Autodesk Inventor part; units mm, degrees
ref_plane "YZ Plane" through (0, 0, 0) normal (1, 0, 0) x (0, 1, 0)
ref_plane "XZ Plane" through (0, 0, 0) normal (0, 1, 0) x (-1, 0, 0)
ref_plane "XY Plane" through (0, 0, 0) normal (0, 0, 1) x (1, 0, 0)
sketch "Boceto1" plane through (0, 0, 0) normal (0, 0, 1) x (1, 0, 0)
  line L0 (-9.55, -9.55) -> (9.55, -9.55)
  line L1 (9.55, -9.55) -> (9.55, 9.55)
  line L2 (9.55, 9.55) -> (-9.55, 9.55)
  line L3 (-9.55, 9.55) -> (-9.55, -9.55)
  line L4 (-9.55, -9.55) -> (9.55, 9.55) construction
  line L5 (9.55, -9.55) -> (-9.55, 9.55) construction
  line L6 (-8.55, 8.55) -> (8.55, 8.55)
  line L7 (8.55, 8.55) -> (8.55, -8.55)
  line L8 (8.55, -8.55) -> (-8.55, -8.55)
  line L9 (-8.55, -8.55) -> (-8.55, 8.55)
  point P0 (0, 0)
  dimension "d0" = 19.1
  dimension "d1" = 19.1
  dimension "d2" = 1
extrude "Extrusión1" add sketch "Boceto1" against normal blind 240
sketch "Boceto2" plane through (-9.55, 9.55, 0) normal (0, 1, 0) x (1, 0, 0)
  line L0 (19.1, 0) -> (0, 0)
  line L1 (9.55, 0) -> (9.55, 240) construction
  line L2 (19.1, 240) -> (0, 240) construction
  point P0 (9.55, 5)
  point P1 (9.55, 30)
  point P2 (9.55, 108)
  point P3 (9.55, 123)
  point P4 (9.55, 138)
  point P5 (9.55, 225)
  point P6 (9.55, 232.75)
  point P7 (9.55, 217.25)
  dimension "d5" = 5
  dimension "d6" = 30
  dimension "d7" = 78
  dimension "d10" = 15
  dimension "d15" = 15
  dimension "d19" = 15.5
  dimension "d24" = 7.75
hole "Agujero1" at (0, 9.55, -5) at (0, 9.55, -30) at (0, 9.55, -108) at (0, 9.55, -123) at (0, 9.55, -138) at (0, 9.55, -217.25) at (0, 9.55, -232.75) direction (0, -1, 0) diameter 3.4 end through all
hole "Agujero2" at (0, 9.55, -225) direction (0, -1, 0) diameter 10 depth 1
sketch "Boceto3" plane through (9.55, -9.55, 0) normal (1, 0, 0) x (0, 0, -1)
  line L0 (240, 19.1) -> (240, 0) construction
  line L1 (240, 9.55) -> (210, 9.55) construction
  circle A0 centre (210, 9.55) radius 5
  point P0 (0, 9.55)
  dimension "d39" = 30
  dimension "d40" = 10
extrude "Extrusión2" cut sketch "Boceto3" against normal up to next
sketch "Boceto4" plane through (9.55, -9.55, 0) normal (1, 0, 0) x (0, 0, -1)
  line L0 (0, 9.55) -> (191.9692, 9.55) construction
  line L1 (0, 0) -> (0, 19.1) construction
  point P0 (100, 9.55)
  point P1 (114, 9.55)
  dimension "d43" = 100
  dimension "d44" = 14
hole "Agujero3" at (9.55, 0, -100) at (9.55, 0, -114) direction (-1, 0, 0) diameter 3.4 end through all
properties part number "perfil" material "Aluminio 6061"
Can you work these out from the model? Positions are in its coordinate system, mm. A direction names the side the tool comes from. Coordinates: 2 decimals unless noted, no trailing zeros. Write each loop counter-clockwise with the first axis right and the second up, starting at its lowest first coordinate (ties: lowest second). Pieces come first, ordered by that corner, then holes. Notation, with made-up numbers: (63.5, 51) - (105.5, 51) arc R24 cw to (105.5, 75) - close; hole circle Ø6 at (69, 6.25). An arc over 180 degrees is marked (long way). Return JSON: item names as keys, results as strings. Group by question number.
Item 1: If we section it at B-B (z = -225): Write out the boundary of the cut face in (x, y).
Item 2: Which directions (+Z, -Z, +X, -X, +Y, -Y) give clear straight access to the entire face, cutting with the end or side of a thin tool? Please do faces 1 (the face through (0, -8.55, -118)), 2 (the face through (-1.5, 9.04, -220.23)), 3 (the face through (9.06, 1.5, -214.77)).
Item 3: Please list where these lines run through material, in increasing order: probe 1 along X at (y, z) = (7.75, -48); probe 2 along X at (y, z) = (-9.3, -138).
Item 4: If we section it at A-A (z = -40.5): Write out the boundary of the cut face in (x, y), then the cut area to 3 significant figures.
Item 5: We'd pull the mould along X, two halves only. Please class faces 4 (the face through (-1, -9, 0)), 5 (the face through (-8.55, 0, -118)), 6 (the face through (-9.55, 0, -118)): pulls with the +X half, pulls with the -X half, needs draft (parallel to the pull), parting line crosses it, or undercut.
Item 6: I'm going to push flat-ended pins straight in: pin 1 Ø4.5 at (y, z) = (0, -114) entering from -X; pin 2 Ø8 at (x, z) = (0, -225) entering from +Y. Where does each tip first touch, or does it pass through?
Return value:
{
 "1": {"outline": "(-9.55, -9.55) - (9.55, -9.55) - (9.55, 9.55) - (5, 9.55) - (5, 8.55) - (8.55, 8.55) - (8.55, -8.55) - (-8.55, -8.55) - (-8.55, 8.55) - (-5, 8.55) - (-5, 9.55) - (-9.55, 9.55) - close"},
 "2": {"face 1": "+Z, -Z", "face 2": "+Y", "face 3": "+X"},
 "3": {"probe 1": "x = -9.55 to -8.55, 8.55 to 9.55", "probe 2": "x = -9.55 to -1.7, 1.7 to 9.55"},
 "4": {"outline": "(-9.55, -9.55) - (9.55, -9.55) - (9.55, 9.55) - (-9.55, 9.55) - close; hole (-8.55, -8.55) - (8.55, -8.55) - (8.55, 8.55) - (-8.55, 8.55) - close", "area": "72.4 mm^2"},
 "5": {"face 4": "needs draft", "face 5": "undercut", "face 6": "pulls with the -X half"},
 "6": {"pin 1": "stops at x = -9.55", "pin 2": "stops at y = -8.55"}
}
